```python
from build123d import *

# Parameters (mm, degrees)
SKETCH2_R           = 1
BOSS_EXTRUDE1_DEPTH = 1
FILLET1_R           = 1.5375


with BuildPart() as part:
    # Sketch2 → Boss-Extrude1 (new body)
    with BuildSketch(Plane.XY):
        with BuildLine():
            Line((3.870772643, -4.941210038), (5.462614208, -6.973265197))
            ThreePointArc((5.462614208, -6.973265197), (7.851985291, 2.288237372), (0, 7.75))
            Line((0, 7.75), (0, 10.25))
            ThreePointArc((0, 10.25), (10.162309829, 1.33789347), (2.652895212, -9.900739719))
            Line((2.652895212, -9.900739719), (1.624559903, -6.062940097))
            Line((1.624559903, -6.062940097), (3.870772643, -4.941210038))
        make_face()
        with Locations((3.663555031, -7.33610009)):
            Circle(SKETCH2_R, mode=Mode.SUBTRACT)
    extrude(amount=BOSS_EXTRUDE1_DEPTH)

    # Fillet1
    fillet1_edges = [part.edges().sort_by_distance(p)[0] for p in [
        (3.870772643, -4.941210038, 0.5),
        (1.624559903, -6.062940097, 0.5),
    ]]
    fillet(fillet1_edges, radius=FILLET1_R - 0.0001)  # a hair under: the kernel refuses the full size

    # Mirror1: part across plane


with BuildPart() as part_1:
    add(part.part)
    add(part.part.mirror(Plane(origin=(0, 10.25, 1), x_dir=(0, 0, 1), z_dir=(1, 0, 0))))


solid = part_1.part
```
Can you work these out from the model? Positions are in its coordinate system, mm. A direction names the side the tool comes from. Coordinates: 2 decimals unless noted, no trailing zeros. Loops run counter-clockwise (first coordinate to the right, second up) from the corner with the lowest first, then second, coordinate; pieces in that order, holes last.
Item 1: Suppose I cut it at C-C (x = -5.75). Please give me the cut outline in (y, z).
Answers below:
outline: (-8.49, 0) - (-6.71, 0) - (-6.71, 1) - (-8.49, 1) - close; (5.46, 0) - (8.49, 0) - (8.49, 1) - (5.46, 1) - close
Item 2: Suppose I cut it at D-D (z = 0.3). State how many separate pieces and enclosed holes the cut face has, then the cut area to 3 significant figures.
Answers below:
separate pieces: 1
enclosed holes: 2
area: 112 mm2
Item 3: I'm going to push flat-ended pins straight in: pin 1 (1.6 mm diameter, centred on x = 3.66, y = -7.34, fed in from +Z); pin 2 (1.5 mm diameter, centred on x = 2, y = 8, fed in from -Z). Where does each tip first touch, or does it pass through?
Answers below:
pin 1: passes through
pin 2: stops at z = 0
Item 4: Suppose I cut it at A-A (y = 2.25). Please give me the cut outline in (x, z).
Answers below:
outline: (-10, 0) - (-7.87, 0) - (-7.87, 1) - (-10, 1) - close; (7.87, 0) - (10, 0) - (10, 1) - (7.87, 1) - close
Item 5: Which directions (+Z, -Z, +X, -X, +Y, -Y) give clear straight access to the entire face, cutting with the end or side of a thin tool? Please do faces 1 (the face through (-2.04, -6.23, 0.51)), 2 (the face through (2.306, -8.606, 0.493)), 3 (the face through (1, 8, 0)).
Answers below:
face 1: +Z, -Z
face 2: +Z, -Z, -Y
face 3: -Z, +X, -X, +Y, -Y
Item 6: Suppose I cut it at B-B (y = -8). Please give me the cut outline in (x, z).
Answers below:
outline: (-6.41, 0) - (-4.41, 0) - (-4.41, 1) - (-6.41, 1) - close; (-2.92, 0) - (-2.14, 0) - (-2.14, 1) - (-2.92, 1) - close; (2.14, 0) - (2.92, 0) - (2.92, 1) - (2.14, 1) - close; (4.41, 0) - (6.41, 0) - (6.41, 1) - (4.41, 1) - close
Item 7: If we mould it in two halves opening along X, with no side actions, what happens to faces 4 (the face through (1, 8, 1)), 5 (the face through (-2.306, -8.606, 0.493))? For each: released by +X, released by -X, zero draft, split by the parting line, or undercut.
Answers below:
face 4: zero draft
face 5: undercut
Item 8: Please list where these lines run through material, in increasing order: L1, parallel to Y at x = -3.25, z = 0.8; L2, parallel to Y at x = -3, z = 0.25; L3, parallel to X at y = -6, z = 0.55.
Answers below:
L1: y = -9.72 to -8.25, -6.43 to -5.35, 7.09 to 9.72
L2: y = -9.8 to -8.08, -6.59 to -5.4, 7.19 to 9.8
L3: x = -8.31 to -6.42, -4.7 to -2.17, 2.17 to 4.7, 6.42 to 8.31
